from build123d import *

# Parameters (mm, degrees)
BOSS_EXTRUDE1_DEPTH      = 1.5
BOSS_EXTRUDE1_DEPTH_BACK = 1.5


with BuildPart() as part:
    # Sketch1 → Boss-Extrude1 (new, two sides: drawn at the far end of the back side and taken through both)
    with BuildSketch(Plane(origin=(0, 0, 0), x_dir=(1, 0, 0), z_dir=(0, 1, 0)).offset(-BOSS_EXTRUDE1_DEPTH_BACK)):
        with BuildLine():
            Line((1.5, -6.837397166), (1.5, -1.3))
            Line((1.5, -1.3), (4.5, -1.3))
            Line((4.5, -1.3), (4.5, 1.3))
            Line((4.5, 1.3), (1.5, 1.3))
            Line((1.5, 1.3), (1.5, 6.837397166))
            ThreePointArc((1.5, 6.837397166), (7, 0), (1.5, -6.837397166))
        make_face()
    extrude(amount=BOSS_EXTRUDE1_DEPTH + BOSS_EXTRUDE1_DEPTH_BACK)


solid = part.part
The model under review builds one solid part; all positions refer to its coordinate system, in mm. A direction names the side the tool comes from. Coordinates: 2 decimals unless noted, no trailing zeros. Write each loop counter-clockwise with the first axis right and the second up, starting at its lowest first coordinate (ties: lowest second). Pieces come first, ordered by that corner, then holes. Notation, with made-up numbers: M 17.5,-18 L 46.5,-18 A17 ccw 46.5,0 Z; hole C -20,-5 d4. An arc over 180 degrees is marked long. Put each result on its own line as item: value.
1) For faces 4 (the flat face through (5, 1.5, 0)), 5 (the flat face through (4.5, 0, 0)), list the 3-axis set-ups (+Z, -Z, +X, -X, +Y, -Y) from which the entire face can be reached by the end or side of a thin tool; tool diameter is ignored.
Computed:
face 4: +Z, -Z, +X, -X, +Y
face 5: -X, +Y, -Y
2) Wall thickness on probe 1 along Z at (x, y) = (3.65, -0.9); probe 2 along Z at (x, y) = (2, -0.7); probe 3 along X at (y, z) = (-0.8, 0): over which ranges is each line inside the solid? List them lowest first. Write a range as [from, to].
Computed:
probe 1: z = [-5.97, -1.3], [1.3, 5.97]
probe 2: z = [-6.71, -1.3], [1.3, 6.71]
probe 3: x = [4.5, 7]
3) Add section D-D on x = 2.4. Give the boundary of the cut face in (y, z), then the cut area to 3 significant figures.
Computed:
outline: M -1.5,-6.58 L 1.5,-6.58 L 1.5,-1.3 L -1.5,-1.3 Z; M -1.5,1.3 L 1.5,1.3 L 1.5,6.58 L -1.5,6.58 Z
area: 31.7 mm2
4) Add section C-C on z = 4.25. Give the boundary of the cut face in (x, y).
Computed:
outline: M 1.5,-1.5 L 5.56,-1.5 L 5.56,1.5 L 1.5,1.5 Z
5) Draft analysis for pull direction Z (two halves, no side actions). For faces 1 (the flat face through (5, -1.5, 0)), 2 (the flat face through (3, 0, -1.3)), 3 (the cylindrical face through (7, 0, 0)), state which applies: released by +Z, released by -Z, zero draft, split by the parting line, or undercut.
Computed:
face 1: zero draft
face 2: undercut
face 3: split by the parting line
6) Add section A-A on x = 4.1. Give the boundary of the cut face in (y, z).
Computed:
outline: M -1.5,-5.67 L 1.5,-5.67 L 1.5,-1.3 L -1.5,-1.3 Z; M -1.5,1.3 L 1.5,1.3 L 1.5,5.67 L -1.5,5.67 Z
7) Add section B-B on y = -0.5. Give the boundary of the cut face in (x, z), then the cut area to 3 significant figures.
Computed:
outline: M 1.5,-6.84 A7 ccw 1.5,6.84 L 1.5,1.3 L 4.5,1.3 L 4.5,-1.3 L 1.5,-1.3 Z
area: 48.3 mm2
8) Clearance check with flat-ended pins moving along their axes: pin 1 Ø1.5 at (x, y) = (5, -1) entering from -Z; pin 2 Ø1.5 at (x, y) = (2.5, 0.5) entering from +Z. State where each tip first meets the part, or that it passes through.
Computed:
pin 1: stops at z = -5.56
pin 2: stops at z = 6.78
